from build123d import *

# Parameters (mm, degrees)
SKETCH_1_W          = 20
SKETCH_1_H          = 15
SKETCH_1_W_2        = 18
SKETCH_1_H_2        = 13
EXTRUDE_1_DEPTH     = 230
SKETCH_3_R          = 1.6
CUT_EXTRUDE_1_DEPTH = 231.989718386
SKETCH_4_R          = 1.6
CUT_EXTRUDE_2_DEPTH = 231.705439901


with BuildPart() as part:
    # 草图1 → 拉伸-薄壁1 (new body)
    with BuildSketch(Plane(origin=(0, 0, 0), x_dir=(1, 0, 0), z_dir=(0, 1, 0))):
        Rectangle(SKETCH_1_W, SKETCH_1_H)
        Rectangle(SKETCH_1_W_2, SKETCH_1_H_2, mode=Mode.SUBTRACT)
    extrude(amount=EXTRUDE_1_DEPTH)

    # 草图3 → 切除-拉伸1 (cut, through all)
    with BuildSketch(Plane(origin=(10, 0, 0), x_dir=(0, 0, -1), z_dir=(1, 0, 0))):
        with Locations((-3.75, 157.5)):
            Circle(SKETCH_3_R)
        with Locations((-3.75, 142.5)):
            Circle(SKETCH_3_R)
        with Locations((3.75, 142.5)):
            Circle(SKETCH_3_R)
        with Locations((3.75, 157.5)):
            Circle(SKETCH_3_R)
        with Locations((-3.75, 87.5)):
            Circle(SKETCH_3_R)
        with Locations((3.75, 87.5)):
            Circle(SKETCH_3_R)
        with Locations((3.75, 72.5)):
            Circle(SKETCH_3_R)
        with Locations((-3.75, 72.5)):
            Circle(SKETCH_3_R)
        with Locations((-3.75, 215)):
            Circle(SKETCH_3_R)
        with Locations((3.75, 215)):
            Circle(SKETCH_3_R)
        with Locations((3.75, 205)):
            Circle(SKETCH_3_R)
        with Locations((-3.75, 205)):
            Circle(SKETCH_3_R)
        with Locations((-3.75, 185)):
            Circle(SKETCH_3_R)
        with Locations((3.75, 185)):
            Circle(SKETCH_3_R)
        with Locations((-3.75, 175)):
            Circle(SKETCH_3_R)
        with Locations((3.75, 175)):
            Circle(SKETCH_3_R)
        with Locations((3.75, 55)):
            Circle(SKETCH_3_R)
        with Locations((-3.75, 55)):
            Circle(SKETCH_3_R)
        with Locations((3.75, 45)):
            Circle(SKETCH_3_R)
        with Locations((-3.75, 45)):
            Circle(SKETCH_3_R)
        with Locations((-3.75, 25)):
            Circle(SKETCH_3_R)
        with Locations((3.75, 25)):
            Circle(SKETCH_3_R)
        with Locations((3.75, 15)):
            Circle(SKETCH_3_R)
        with Locations((-3.75, 15)):
            Circle(SKETCH_3_R)
    extrude(amount=-CUT_EXTRUDE_1_DEPTH, mode=Mode.SUBTRACT)

    # 草图4 → 切除-拉伸2 (cut, through all)
    with BuildSketch(Plane(origin=(0, 0, -7.5), x_dir=(-1, 0, 0), z_dir=(0, 0, -1))):
        with Locations((5, 225)):
            Circle(SKETCH_4_R)
        with Locations((-5, 225)):
            Circle(SKETCH_4_R)
        with Locations((5, 215)):
            Circle(SKETCH_4_R)
        with Locations((-5, 215)):
            Circle(SKETCH_4_R)
        with Locations((-5, 195)):
            Circle(SKETCH_4_R)
        with Locations((5, 195)):
            Circle(SKETCH_4_R)
        with Locations((-5, 185)):
            Circle(SKETCH_4_R)
        with Locations((5, 185)):
            Circle(SKETCH_4_R)
        with Locations((-5, 165)):
            Circle(SKETCH_4_R)
        with Locations((5, 165)):
            Circle(SKETCH_4_R)
        with Locations((-5, 155)):
            Circle(SKETCH_4_R)
        with Locations((5, 155)):
            Circle(SKETCH_4_R)
        with Locations((-5, 135)):
            Circle(SKETCH_4_R)
        with Locations((5, 135)):
            Circle(SKETCH_4_R)
        with Locations((-5, 125)):
            Circle(SKETCH_4_R)
        with Locations((5, 125)):
            Circle(SKETCH_4_R)
        with Locations((-5, 105)):
            Circle(SKETCH_4_R)
        with Locations((5, 105)):
            Circle(SKETCH_4_R)
        with Locations((-5, 95)):
            Circle(SKETCH_4_R)
        with Locations((5, 95)):
            Circle(SKETCH_4_R)
        with Locations((-5, 75)):
            Circle(SKETCH_4_R)
        with Locations((5, 75)):
            Circle(SKETCH_4_R)
        with Locations((-5, 65)):
            Circle(SKETCH_4_R)
        with Locations((5, 65)):
            Circle(SKETCH_4_R)
        with Locations((-5, 45)):
            Circle(SKETCH_4_R)
        with Locations((5, 45)):
            Circle(SKETCH_4_R)
        with Locations((-5, 35)):
            Circle(SKETCH_4_R)
        with Locations((5, 35)):
            Circle(SKETCH_4_R)
        with Locations((-5, 15)):
            Circle(SKETCH_4_R)
        with Locations((5, 15)):
            Circle(SKETCH_4_R)
        with Locations((-5, 5)):
            Circle(SKETCH_4_R)
        with Locations((5, 5)):
            Circle(SKETCH_4_R)
    extrude(amount=-CUT_EXTRUDE_2_DEPTH, mode=Mode.SUBTRACT)


solid = part.part
Can you work these out from the model? Positions are in its coordinate system, mm. A direction names the side the tool comes from. Give positions to 0.01 mm unless a question says otherwise; leave off trailing zeros. One line per item, written item: value. Start each with the question number.
1) On a 3-axis mill with a long thin cutter (end or side, diameter ignored), from which of +Z, -Z, +X, -X, +Y, -Y can I reach the whole of each face in a straight line? I mean faces 1 (the face through (-1, 230, 7)), 2 (the face through (-9, 113, 0)). Say none if no direction works.
2) I'm going to push a flat-ended pin straight in: pin 1 (1.9 mm diameter, centred on y = 15, z = -3.75, fed in from -X). Where does the tip first touch, or does it pass through?
3) Thinking about a two-plate mould opening in X: for faces 3 (the face through (0, 113, -6.5)), 4 (the face through (10, 113, 0)), 5 (the face through (0, 113, -7.5)), which applies, +X half, -X half, draft (parallel to the pull), parting line (faces both ways), or undercut?
4) If I drill on line 1 (Z direction, x = -9.5, y = 72.5); line 2 (X direction, y = 110, z = -0.5); line 3 (X direction, y = 195, z = 7.15), over which ranges is the centre line in solid material (lowest first)? Write a range as [from, to].
Completed:
1. face 1: +Z, -Z, +X, -X, +Y
1. face 2: +Y, -Y
2. pin 1: passes through
3. face 3: undercut
3. face 4: +X half
3. face 5: draft
4. line 1: z = [-7.5, -5.35], [-2.15, 2.15], [5.35, 7.5]
4. line 2: x = [-10, -9], [9, 10]
4. line 3: x = [-10, -6.6], [-3.4, 3.4], [6.6, 10]
